```python
from build123d import *

# Parameters (mm, degrees)
SKETCH_4_W      = 56
SKETCH_4_H      = 40
EXTRUDE_2_DEPTH = 8.8
SKETCH_5_W      = 8.8
SKETCH_5_H      = 13.2
EXTRUDE_3_DEPTH = 40


with BuildPart() as part:
    # 스케치4 → 보스-돌출2 (new body)
    with BuildSketch(Plane(origin=(0, 0, 0), x_dir=(1, 0, 0), z_dir=(0, 1, 0))):
        with Locations((28, 20)):
            Rectangle(SKETCH_4_W, SKETCH_4_H)
    extrude(amount=EXTRUDE_2_DEPTH)

    # 스케치5 → 보스-돌출3 (add)
    with BuildSketch(Plane.XY):
        Polygon((0, 8.8), (0, 32), (3.2, 32), (16.594526245, 8.8), align=None)
        with Locations((51.6, 15.4)):
            Rectangle(SKETCH_5_W, SKETCH_5_H)
    extrude(amount=-EXTRUDE_3_DEPTH)


solid = part.part
```
Could you check a few things on this model? Use its own coordinates, in mm. A direction names the side the tool comes from. Give positions to 0.01 mm unless a question says otherwise; leave off trailing zeros. Loops run counter-clockwise (first coordinate to the right, second up) from the corner with the lowest first, then second, coordinate; pieces in that order, holes last. Notation, with made-up numbers: (-2, 1.5) - (15, 1.5) arc R26 cw to (15, 36.5) - close; hole circle Ø1 at (7, 42.25). An arc over 180 degrees is marked (long way). Use one line per item in the form item = value.
1. I want a section at C-C (x = 39.5). Please give me the cut outline in (y, z).
Response values:
outline = (0, -40) - (8.8, -40) - (8.8, 0) - (0, 0) - close
2. I need wall thicknesses on probe 1 along Y at (x, z) = (19, -19.5); probe 2 along X at (y, z) = (14.5, -23); probe 3 along X at (y, z) = (13, -7). Which ranges of each line are inside material? Lowest first, please.
Response values:
probe_1 = 0 to 8.8
probe_2 = 0 to 13.3, 47.2 to 56
probe_3 = 0 to 14.17, 47.2 to 56
3. I want a section at A-A (y = 11). Please give me the cut outline in (x, z).
Response values:
outline = (0, -40) - (15.32, -40) - (15.32, 0) - (0, 0) - close; (47.2, -40) - (56, -40) - (56, 0) - (47.2, 0) - close
4. On a 3-axis mill with a long thin cutter (end or side, diameter ignored), from which of +Z, -Z, +X, -X, +Y, -Y can I reach the whole of each face in a straight line? I mean faces 4 (the face through (32, 8.8, -20)), 5 (the face through (22, 6, -40)), 6 (the face through (52, 22, -20)). Say none if no direction works.
Response values:
face_4 = +Z, -Z, +Y
face_5 = -Z, +X, -X, +Y, -Y
face_6 = +Z, -Z, +X, +Y
5. I want a section at B-B (z = -32). Please give me the cut outline in (x, y).
Response values:
outline = (0, 0) - (56, 0) - (56, 22) - (47.2, 22) - (47.2, 8.8) - (16.59, 8.8) - (3.2, 32) - (0, 32) - close
6. Thinking about a two-plate mould opening in X: for faces 1 (the face through (0, 16, -20)), 2 (the face through (2, 32, -20)), 3 (the face through (47.2, 15, -20)), which applies, released by +X, released by -X, zero draft, split by the parting line, or undercut?
Response values:
face_1 = released by -X
face_2 = zero draft
face_3 = undercut
7. I want a section at D-D (y = 16). Please give me the cut outline in (x, z).
Response values:
outline = (0, -40) - (12.44, -40) - (12.44, 0) - (0, 0) - close; (47.2, -40) - (56, -40) - (56, 0) - (47.2, 0) - close
8. I'm going to push flat-ended pins straight in: pin 1 Ø1 at (x, z) = (5.5, -18) entering from +Y; pin 2 Ø7 at (x, z) = (51, -18.5) entering from +Y; pin 3 Ø2 at (x, z) = (16, -34.5) entering from -Y; pin 4 Ø6 at (x, z) = (42, -28) entering from +Y. Where does each tip first touch, or does it pass through?
Response values:
pin_1 = 28.88
pin_2 = 22
pin_3 = 0
pin_4 = 8.8
